Input: part model. Units: mm. Frame: model coordinates. Face numbers are marked on the shaded views. A direction names the side the tool comes from. Coordinates: 2 decimals unless noted, no trailing zeros. Order: outer loops, then holes, each group sorted by start corner. A loop starts at its lowest first (then second) coordinate and runs counter-clockwise, first axis right, second up.
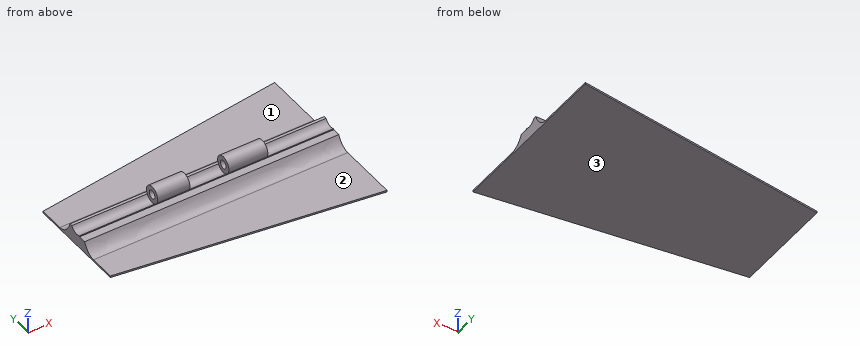
from build123d import *

# Parameters (mm, degrees)
BOSS_EXTRUDE1_DEPTH      = 1
BOSS_EXTRUDE5_DEPTH      = 100
BOSS_EXTRUDE5_DEPTH_BACK = 1
SKETCH2_W                = 214
SKETCH2_H                = 10
FILLET3_SIZE             = 15
FILLET3_SIZE_2           = 10
CUT_EXTRUDE2_DEPTH       = 229
SKETCH7_W                = 64
SKETCH7_H                = 10
CUT_EXTRUDE3_DEPTH       = 14
EXTRUDE_THIN2_START      = -40.5
SKETCH9_R                = 5
SKETCH9_R_2              = 2.5
EXTRUDE_THIN2_DEPTH      = 23
EXTRUDE_THIN3_START      = -86.5
SKETCH9_3_R              = 5
SKETCH9_3_R_2            = 2.5
EXTRUDE_THIN3_DEPTH      = 19
CUT_EXTRUDE8_DEPTH       = 71
CUT_EXTRUDE8_DEPTH_BACK  = 153


with BuildPart() as part:
    # Sketch1 → Boss-Extrude1 (new body)
    with BuildSketch(Plane.XY):
        Polygon((75, 50), (75, -50), (-75, -30), (-75, 30), align=None)
    extrude(amount=BOSS_EXTRUDE1_DEPTH)

    # Sketch2 → Boss-Extrude5 (add, two sides: drawn at the far end of the back side and taken through both)
    with BuildSketch(Plane.XY.offset(1).offset(-BOSS_EXTRUDE5_DEPTH_BACK)):
        with Locations((32, 0)):
            Rectangle(SKETCH2_W, SKETCH2_H)
    extrude(amount=BOSS_EXTRUDE5_DEPTH + BOSS_EXTRUDE5_DEPTH_BACK)

    # Fillet3
    # an asymmetric fillet: 15, 10 mm, written as the material it adds along each edge
    with BuildSketch(Plane(origin=(75, -5, 1), x_dir=(0, 0, 1), z_dir=(-1, 0, 0))) as fillet3_piece_1:
        with BuildLine():
            Bezier((FILLET3_SIZE, 0), (0, 0), (0, -FILLET3_SIZE_2), weights=[1, 0.707106781, 1])
            Line((0, -FILLET3_SIZE_2), (0, 0))
            Line((0, 0), (FILLET3_SIZE, 0))
        make_face()
    extrude(amount=150)
    with BuildSketch(Plane(origin=(-75, 5, 1), x_dir=(0, 1, 0), z_dir=(1, 0, 0))) as fillet3_piece_2:
        with BuildLine():
            Bezier((FILLET3_SIZE_2, 0), (0, 0), (0, FILLET3_SIZE), weights=[1, 0.707106781, 1])
            Line((0, FILLET3_SIZE), (0, 0))
            Line((0, 0), (FILLET3_SIZE_2, 0))
        make_face()
    extrude(amount=150)

    # Sketch6 → Cut-Extrude2 (cut)
    with BuildSketch(Plane.ZY.offset(75)):
        with BuildLine():
            Line((9.5, 6.986773712), (9.5, 4.330127019))
            ThreePointArc((9.5, 4.330127019), (7, 0), (9.5, -4.330127019))
            Line((9.5, -4.330127019), (9.5, -7.297871365))
            Line((9.5, -7.297871365), (14.5, -7.297871365))
            Line((14.5, -7.297871365), (14.5, -4.330127019))
            ThreePointArc((14.5, -4.330127019), (17, 0), (14.5, 4.330127019))
            Line((14.5, 4.330127019), (14.5, 6.986773712))
            Line((14.5, 6.986773712), (9.5, 6.986773712))
        make_face()
    extrude(amount=-CUT_EXTRUDE2_DEPTH, mode=Mode.SUBTRACT)


with BuildPart() as cut_extrude2_piece_1:
    # of the separate pieces the step leaves, piece 1, a body of its own (cut_extrude2_pieces)
    add(part.part.solids().sort_by_distance((-75, 5.050125629, 14.5))[0])


with BuildPart() as cut_extrude2_piece_2:
    # of the separate pieces the step leaves, piece 2, a body of its own (cut_extrude2_pieces)
    add(part.part.solids().sort_by_distance((-75, 15, 1))[0])

    # Sketch7 → Cut-Extrude3 (cut)
    with BuildSketch(Plane(origin=(0, 0, 0), x_dir=(-1, 0, 0), z_dir=(0, 0, -1))):
        with Locations((-107, 0)):
            Rectangle(SKETCH7_W, SKETCH7_H)
    extrude(amount=-CUT_EXTRUDE3_DEPTH, mode=Mode.SUBTRACT)

    # Sketch9 → Extrude-Thin2 (add)
    with BuildSketch(Plane(origin=(75, 0, 0), x_dir=(0, 0, -1), z_dir=(1, 0, 0)).offset(EXTRUDE_THIN2_START)):
        with Locations((-12, 0)):
            Circle(SKETCH9_R)
        with Locations((-12, 0)):
            Circle(SKETCH9_R_2, mode=Mode.SUBTRACT)
    extrude(amount=-EXTRUDE_THIN2_DEPTH)

    # Sketch9<3> → Extrude-Thin3 (add)
    with BuildSketch(Plane(origin=(75, 0, 0), x_dir=(0, 0, -1), z_dir=(1, 0, 0)).offset(EXTRUDE_THIN3_START)):
        with Locations((-12, 0)):
            Circle(SKETCH9_3_R)
        with Locations((-12, 0)):
            Circle(SKETCH9_3_R_2, mode=Mode.SUBTRACT)
    extrude(amount=-EXTRUDE_THIN3_DEPTH)

    # Sketch12 → Cut-Extrude8 (cut, two sides: drawn at the far end of the back side and taken through both)
    with BuildSketch(Plane.ZY.offset(30.5).offset(-CUT_EXTRUDE8_DEPTH_BACK)):
        with BuildLine():
            Line((7, -2.5), (7.669872981, -2.5))
            ThreePointArc((7.669872981, -2.5), (8.464466094, -3.535533906), (9.5, -4.330127019))
            Line((9.5, -4.330127019), (9.5, -7.690384485))
            Line((9.5, -7.690384485), (7, -7.690384485))
            Line((7, -7.690384485), (7, -2.5))
        make_face()
    extrude(amount=CUT_EXTRUDE8_DEPTH + CUT_EXTRUDE8_DEPTH_BACK, mode=Mode.SUBTRACT)


solid = cut_extrude2_piece_2.part
Item 1: Cut plane B-B on z = 12. Return loops of the section in (x, y).
Response values:
outline: (-30.5, -5) - (-11.5, -5) - (-11.5, -2.5) - (-30.5, -2.5) - close; (-30.5, 2.5) - (-11.5, 2.5) - (-11.5, 5) - (-30.5, 5) - close; (11.5, -5) - (34.5, -5) - (34.5, -2.5) - (11.5, -2.5) - close; (11.5, 2.5) - (34.5, 2.5) - (34.5, 5) - (11.5, 5) - close
Item 2: Ray query, probe 1 along Y at (x, z) = (-16.25, 12); probe 2 along Z at (x, y) = (23, 14.5); probe 3 along Y at (x, z) = (40, 2.5). Return the intervals inside material, ascending.
Response values:
probe 1: y = -5 to -2.5, 2.5 to 5
probe 2: z = 0 to 1.02
probe 3: y = -10.64 to 10.64
Item 3: Cut plane A-A on y = 0. Return loops of the section in (x, z).
Response values:
outline: (-75, 0) - (75, 0) - (75, 7) - (34.5, 7) - (34.5, 9.5) - (11.5, 9.5) - (11.5, 7) - (-11.5, 7) - (-11.5, 9.5) - (-30.5, 9.5) - (-30.5, 7) - (-75, 7) - close; (-30.5, 14.5) - (-11.5, 14.5) - (-11.5, 17) - (-30.5, 17) - close; (11.5, 14.5) - (34.5, 14.5) - (34.5, 17) - (11.5, 17) - close
Item 4: Pin query (flat end, axial travel): pin 1 Ø0.8 at (x, y) = (0.5, 5) entering from +Z; pin 2 Ø17.5 at (x, y) = (28, 33.5) entering from +Z; pin 3 Ø5 at (y, z) = (0.5, 10.5) entering from -X; pin 4 Ø8 at (x, y) = (55, -29.5) entering from -Z. Return the tip coordinate at first contact, or that it passes through.
Response values:
pin 1: stops at z = 9.5
pin 2: stops at z = 1
pin 3: stops at x = -30.5
pin 4: stops at z = 0
Item 5: Access query for the marked faces 1, 2 and 3. Directions: +Z, -Z, +X, -X, +Y, -Y. A direction counts if a zero-diameter tool reaches every point of the face in a straight line with its end or side. Return the directions, or none.
Response values:
face 1: +Z, +X, -X, +Y
face 2: +Z, +X, -X, -Y
face 3: -Z, +X, -X, +Y, -Y
